Could you check a few things on this model? Use its own coordinates, in mm. A direction names the side the tool comes from. Coordinates: 2 decimals unless noted, no trailing zeros. Write each loop counter-clockwise with the first axis right and the second up, starting at its lowest first coordinate (ties: lowest second). Pieces come first, ordered by that corner, then holes.
Item 1: I want a section at A-A on z = -5.5. Please give me the cut outline in (x, y), then the cut area to 3 significant figures.
Item 2: I want a section at B-B on x = 5. Please give me the cut outline in (y, z).
Item 3: I want a section at D-D on z = 20.5. Please give me the cut outline in (x, y), then the cut area to 3 significant figures.
Item 4: Which directions (+Z, -Z, +X, -X, +Y, -Y) give clear straight access to the entire face, cutting with the end or side of a thin tool? Please do faces 1 (the cylindrical face through (0.1, -1.26, -17.06)), 2 (the cylindrical face through (0.1, -2.53, 17.55)), 3 (the cylindrical face through (0.1, -3.4, -18.05)).
Item 5: If I drill on probe 1 along Z at (x, y) = (-1.5, 7.5); probe 2 along Y at (x, z) = (3.25, -10.5); probe 3 along Z at (x, y) = (2.25, 6), over which ranges is the centre line in solid material (lowest first)?
Item 6: For P1, Ø6, axis at x = -4, z = 4.5, coming from the +Y side; P2, Ø1.5, axis at x = -0.5, y = -1, coming from the +Z side; P3, Ø6, axis at x = -1.5, y = 7, coming from the -Z side, each with a flat end and sliding along its axis, tell me the tip position at first contact or that it passes through.
Item 7: I want a section at C-C on y = 2. Please give me the cut outline in (x, z), then the cut area to 3 significant figures.
Item 8: Thinking about a two-plate mould opening in Y: for faces 4 (the cylindrical face through (0.098, 10.216, 21.181)), 5 (the cylindrical face through (0.098, 9.265, 20.851)), 6 (the flat face through (-7, -2, 0)), which applies, +Y half, -Y half, draft (parallel to the pull), parting line (faces both ways), or undercut?
from build123d import *

# Parameters (mm, degrees)
BOSS_EXTRUDE1_DEPTH = 7


with BuildPart() as part:
    # Sketch1 → Boss-Extrude1 (new body, symmetric)
    with BuildSketch(Plane(origin=(0, 0, 0), x_dir=(0, 0, -1), z_dir=(1, 0, 0))):
        with BuildLine():
            Line((-22.14614181, 6.771839894), (-18.561151485, -1.33269977))
            ThreePointArc((-18.561151485, -1.33269977), (-17.528308744, -2.546439623), (-16.000496078, -3))
            Line((-16.000496078, -3), (0, -3))
            Line((0, -3), (0, -4))
            Line((0, -4), (-16.000496078, -4))
            ThreePointArc((-16.000496078, -4), (-18.073958177, -3.384453165), (-19.475674713, -1.737233163))
            Line((-19.475674713, -1.737233163), (-23.060665038, 6.367306501))
            ThreePointArc((-23.060665038, 6.367306501), (-21.114031535, 10.231842835), (-17.700926013, 7.572005665))
            Line((-17.700926013, 7.572005665), (-17.5, -0.238584995))
            ThreePointArc((-17.5, -0.238584995), (-17.047428938, -1.274222609), (-16.000495091, -1.700010532))
            Line((-16.000495091, -1.700010532), (0, -1.7))
            Line((0, -1.7), (0, -2.7))
            Line((0, -2.7), (-16.000494433, -2.700010532))
            ThreePointArc((-16.000494433, -2.700010532), (-17.745384177, -1.990363995), (-18.499669281, -0.264301304))
            Line((-18.499669281, -0.264301304), (-18.700595294, 7.546289356))
            ThreePointArc((-18.700595294, 7.546289356), (-20.894734558, 9.25618468), (-22.14614181, 6.771839894))
        make_face()
    boss_extrude1 = extrude(amount=BOSS_EXTRUDE1_DEPTH, both=True)

    # Mirror1: Boss-Extrude1 across plane
    add(boss_extrude1.mirror(Plane.XY))


solid = part.part
Response values:
1. outline: (-7, -4) - (7, -4) - (7, -3) - (-7, -3) - close; (-7, -2.7) - (7, -2.7) - (7, -1.7) - (-7, -1.7) - close
1. area: 28.0 mm2
2. outline: (-4, -16) arc R3.8 ccw to (-1.74, -19.48) - (6.37, -23.06) arc R2.8 ccw (long way) to (7.57, -17.7) - (-0.24, -17.5) arc R1.5 cw to (-1.7, -16) - (-1.7, 0) - (-1.7, 16) arc R1.5 cw to (-0.24, 17.5) - (7.57, 17.7) arc R2.8 ccw (long way) to (6.37, 23.06) - (-1.74, 19.48) arc R3.8 ccw to (-4, 16) - close; hole (-3, -16) arc R2.8 ccw to (-1.33, -18.56) - (6.77, -22.15) arc R1.8 ccw (long way) to (7.55, -18.7) - (-0.26, -18.5) arc R2.5 cw to (-2.7, -16) - (-2.7, 0) - (-2.7, 16) arc R2.5 cw to (-0.26, 18.5) - (7.55, 18.7) arc R1.8 ccw (long way) to (6.77, 22.15) - (-1.33, 18.56) arc R2.8 ccw to (-3, 16) - close
3. outline: (-7, 0.58) - (7, 0.58) - (7, 3.05) - (-7, 3.05) - close; (-7, 9.3) - (7, 9.3) - (7, 10.3) - (-7, 10.3) - close
3. area: 48.6 mm2
4. face 1: +X, -X, +Y
4. face 2: +X, -X
4. face 3: -Z, +X, -X, -Y
5. probe 1: z = -23.3 to -22.3, -18.7 to -17.7, 17.7 to 18.7, 22.3 to 23.3
5. probe 2: y = -4 to -3, -2.7 to -1.7
5. probe 3: z = -22.9 to -21.8, -18.66 to -17.66, 17.66 to 18.66, 21.8 to 22.9
6. P1: stops at y = -1.7
6. P2: stops at z = 20.13
6. P3: stops at z = -23.3
7. outline: (-7, -21.13) - (7, -21.13) - (7, -20.04) - (-7, -20.04) - close; (-7, -18.56) - (7, -18.56) - (7, -17.56) - (-7, -17.56) - close; (-7, 17.56) - (7, 17.56) - (7, 18.56) - (-7, 18.56) - close; (-7, 20.04) - (7, 20.04) - (7, 21.13) - (-7, 21.13) - close
7. area: 58.6 mm2
8. face 4: parting line
8. face 5: undercut
8. face 6: draft
